Verification items for the finished model (mm, model axes). A direction names the side the tool comes from. Round coordinates to 2 decimals unless told otherwise and drop trailing zeros. Write each loop counter-clockwise with the first axis right and the second up, starting at its lowest first coordinate (ties: lowest second). Pieces come first, ordered by that corner, then holes. Notation, with made-up numbers: M -16.75,64 L 12.25,64 A4 cw 12.25,70 Z; hole C 1.5,24 d11. An arc over 180 degrees is marked long. Answer in a Markdown table with one row per item. Add a question column.
1. Set-up check for faces 1 (the flat face through (-15, 38, 0)), 2 (the cylindrical face through (-8.57, 45.39, 1.01)): record each of +Z, -Z, +X, -X, +Y, -Y from which the full face is reachable in a straight line by a thin tool's end or side.
2. Draft check along X on faces 3 (the flat face through (-31.52, 47.32, 0.99)), 4 (the cylindrical face through (-43.968, 106.947, 0.986)), 5 (the cylindrical face through (-35.71, 78.51, 1.01)). Enter one of: pulls with the +X half, pulls with the -X half, needs draft (parallel to the pull), parting line crosses it, or undercut.
3. Sectioned sample at A-A on x = -42. Record the cut outline in (y, z), plus the area to 3 significant figures.
4. Sectioned sample at C-C on z = 0.9. Count the separate pieces of the cut face and the enclosed holes in it, plus the area to 3 significant figures.
5. Material ranges on probe 1 along Y at (x, z) = (9, 0.45); probe 2 along X at (y, z) = (61, 1.9); probe 3 along Y at (x, z) = (-14.5, 1.15), recorded low to high.
6. Go/stop test with a flat-tipped pin: pin 1 Ø3.5 at (x, y) = (-17.72, 60.66) entering from +Z. Record where the tip stops, or that it passes through.
7. Sectioned sample at D-D on x = 2. Record the cut outline in (y, z), plus the area to 3 significant figures.
8. Sectioned sample at B-B on y = 72.5. Record the cut outline in (x, z).
Autodesk Inventor part; units mm, degrees
ref_plane "YZ Plane" through (0, 0, 0) normal (1, 0, 0) x (0, 1, 0)
ref_plane "XZ Plane" through (0, 0, 0) normal (0, 1, 0) x (-1, 0, 0)
ref_plane "XY Plane" through (0, 0, 0) normal (0, 0, 1) x (1, 0, 0)
sketch "Эскиз1" plane through (0, 0, 0) normal (0, 0, 1) x (1, 0, 0)
  line L0 (15, -22.25) -> (15, 22.25)
  line L1 (15, 22.25) -> (-20, 22.25)
  line L2 (-20, 22.25) -> (-20, -22.25)
  line L3 (-20, -22.25) -> (15, -22.25)
  circle A0 centre (8.763, 2.3275) radius 1.5
  circle A1 centre (8.763, 7.3275) radius 1.5
  circle A2 centre (-11.237, -7.6725) radius 1.5
  circle A3 centre (-11.237, -2.6725) radius 1.5
  circle A4 centre (8.763, -2.6725) radius 1.5
  circle A5 centre (8.763, -7.6725) radius 1.5
  circle A6 centre (-11.237, 2.3275) radius 1.5
  circle A7 centre (-11.237, 7.3275) radius 1.5
  line L4 (-25, 92.25) -> (-62.0049, 92.25)
  line L5 (-103.637, 92.25) -> (-67.893, 92.25)
  circle A8 centre (-49, 104.25) radius 1.5
  circle A9 centre (-42, 104.25) radius 1.5
  circle A10 centre (-35, 104.25) radius 1.5
  circle A11 centre (-35, 111.25) radius 1.5
  circle A12 centre (-42, 118.25) radius 1.5
  circle A13 centre (-49, 118.25) radius 1.5
  circle A14 centre (-49, 111.25) radius 1.5
  circle A15 centre (-35, 118.25) radius 1.5
  circle A16 centre (-42, 111.25) radius 1.5
  circle A17 centre (-42, 97.25) radius 1.5
  circle A18 centre (-35, 97.25) radius 1.5
  circle A19 centre (-49, 97.25) radius 1.5
  line L6 (-25, 92.25) -> (-62.0049, 92.25)
  line L7 (-25, 95.25) -> (-25, 92.25)
  line L8 (-20, 95.25) -> (-25, 95.25)
  line L9 (-20, 95.25) -> (-20, 123.25)
  line L10 (-28, 123.25) -> (-20, 123.25)
  line L11 (-28, 129.25) -> (-28, 123.25)
  line L12 (-28, 129.25) -> (-62.0049, 129.25)
  line L13 (-62.0049, 92.25) -> (-62.0049, 129.25)
  line L14 (-5.1452, 11.625) -> (-40, 100) construction
  arc A20 (-32.5697, 102.9649) -> (-47.4303, 97.0351) centre (-40, 100) ccw
  line L15 (-5.1452, 11.625) -> (-22.5726, 55.8125) construction
  arc A21 (-13.8135, 8.0713) -> (-4.3725, 15.1785) centre (-0.8009, 0.6099) ccw
  line L16 (12.7625, 7.0157) -> (-32.7662, 103.4164)
  line L17 (-47.6184, 97.5588) -> (-15.0854, -3.9674)
  point P0 (0, 0)
  point P1 (-13.8589, 33.7187)
  point P2 (-33.6095, 104.8127)
  point P3 (-34.2206, 105.5316)
  point P4 (-47.7749, 98.1155)
  point P5 (-47.5011, 97.1926)
  dimension "d0" = 8
  dimension "d1" = 95
  dimension "d2" = 100
  dimension "d3" = 40
  dimension "d4" = 15
extrude "Выдавливание1" add sketch "Эскиз1" along normal blind 2 contours L16 A21 L17 L2 L1 | L1 L2 L17 L4 L16 | L4 L17 A19 A20 A10 L16 | A20 A10 | A10 A20 | A1 | A2 | A3 | A4 | A5 | A7 | A9
sketch "Эскиз2" plane through (0, 0, 2) normal (0, 0, 1) x (1, 0, 0)
  circle A0 centre (-38.5661, 86.5462) radius 1.5
  line L0 (-47.5011, 97.1926) -> (-15.0854, -3.9674)
  circle A1 centre (-35.5146, 77.0232) radius 1.5
  circle A2 centre (-32.463, 67.5001) radius 1.5
  circle A3 centre (-29.4114, 57.9771) radius 1.5
  circle A4 centre (-26.3599, 48.4541) radius 1.5
  circle A5 centre (-23.3083, 38.9311) radius 1.5
  circle A6 centre (-20.2568, 29.408) radius 1.5
  circle A7 centre (-17.2052, 19.885) radius 1.5
  circle A8 centre (-42, 97.25) radius 1.5
  circle A9 centre (-11.237, 2.3275) radius 1.5
  point P0 (0, 0)
  dimension "d7" = 3
  dimension "d10" = 10
  dimension "d17" = 5.2562
  dimension "d18" = 5.26
extrude "Выдавливание2" cut sketch "Эскиз2" against normal blind 3 contours A0 | A1 | A2 | A3 | A4 | A5 | A6 | A7
sketch "Эскиз3" plane through (0, 0, 2) normal (0, 0, 1) x (1, 0, 0)
  circle A0 centre (-35, 97.25) radius 1.5
  line L0 (12.7625, 7.0157) -> (-32.7662, 103.4164)
  circle A1 centre (-30.5318, 87.7899) radius 1.5
  circle A2 centre (-26.2613, 78.7476) radius 1.5
  circle A3 centre (-21.9908, 69.7054) radius 1.5
  circle A4 centre (-17.7202, 60.6631) radius 1.5
  circle A5 centre (-13.4497, 51.6208) radius 1.5
  circle A6 centre (-9.1792, 42.5786) radius 1.5
  circle A7 centre (-4.9086, 33.5363) radius 1.5
  circle A8 centre (-0.6381, 24.494) radius 1.5
  point P0 (0, 0)
  dimension "d19" = 3
  dimension "d20" = 4.6533
  dimension "d21" = 4.653
  dimension "d24" = 10
extrude "Выдавливание3" cut sketch "Эскиз3" against normal blind 3 contours A1 | A2 | A3 | A4 | A5 | A6 | A7 | A8
sketch "Эскиз4" plane through (0, 0, 0) normal (0, 0, -1) x (-1, 0, 0)
  circle A0 centre (42, 97.25) radius 1.5
  circle A1 centre (35, 97.25) radius 1.5
  arc A2 (35, 97.25) -> (36.2942, 93.1949) centre (42, 97.25) ccw construction
  arc A3 (33.5, 97.25) -> (35.0715, 92.326) centre (42, 97.25) ccw
  arc A4 (36.5, 97.25) -> (37.5169, 94.0639) centre (42, 97.25) ccw
  arc A5 (36.5, 97.25) -> (33.5, 97.25) centre (35, 97.25) ccw
  arc A6 (35.0715, 92.326) -> (37.5169, 94.0639) centre (36.2942, 93.1949) ccw
  point P0 (0, 0)
extrude "Выдавливание4" cut sketch "Эскиз4" against normal blind 3 contours A4 A6 A3 A1
sketch "Эскиз5" plane through (0, 0, 2) normal (0, 0, 1) x (1, 0, 0)
  circle A0 centre (-42, 97.25) radius 1.5
  arc A1 (-35.0715, 92.326) -> (-33.5, 97.25) centre (-42, 97.25) ccw
  arc A2 (-37.5169, 94.0639) -> (-35.0715, 92.326) centre (-36.2942, 93.1949) ccw
  arc A3 (-37.5169, 94.0639) -> (-36.5, 97.25) centre (-42, 97.25) ccw
  arc A4 (-33.5, 97.25) -> (-36.5, 97.25) centre (-35, 97.25) ccw
  circle A5 centre (-11.237, 2.3275) radius 1.5
  circle A6 centre (8.763, 2.3275) radius 1.5
  arc A7 (-15.0854, -3.9674) -> (12.7625, 7.0157) centre (-0.8009, 0.6099) ccw
  line L0 (12.7625, 7.0157) -> (-32.7662, 103.4164)
  arc A8 (-32.7662, 103.4164) -> (-33.6095, 104.8127) centre (-40, 100) ccw
  arc A9 (-33.6095, 104.8127) -> (-34.2206, 105.5316) centre (-35, 104.25) ccw
  arc A10 (-34.2206, 105.5316) -> (-47.7749, 98.1155) centre (-40, 100) ccw
  arc A11 (-47.5011, 97.1926) -> (-47.7749, 98.1155) centre (-49, 97.25) ccw
  line L1 (-47.5011, 97.1926) -> (-15.0854, -3.9674)
  circle A12 centre (-17.2052, 19.885) radius 1.5
  circle A13 centre (-23.3083, 38.9311) radius 1.5
  circle A14 centre (-38.5661, 86.5462) radius 1.5
  circle A15 centre (-32.463, 67.5001) radius 1.5
  circle A16 centre (-29.4114, 57.9771) radius 1.5
  circle A17 centre (-35.5146, 77.0232) radius 1.5
  circle A18 centre (-20.2568, 29.408) radius 1.5
  circle A19 centre (-26.3599, 48.4541) radius 1.5
  circle A20 centre (-0.6381, 24.494) radius 1.5
  circle A21 centre (-26.2613, 78.7476) radius 1.5
  circle A22 centre (-4.9086, 33.5363) radius 1.5
  circle A23 centre (-13.4497, 51.6208) radius 1.5
  circle A24 centre (-17.7202, 60.6631) radius 1.5
  circle A25 centre (-9.1792, 42.5786) radius 1.5
  circle A26 centre (-30.5318, 87.7899) radius 1.5
  circle A27 centre (-21.9908, 69.7054) radius 1.5
  circle A28 centre (-23.3083, 38.9311) radius 1.5
  circle A29 centre (-9.1792, 42.5786) radius 1.5
  arc A30 (-9.149, 35.4026) -> (-9.1792, 42.5786) centre (-23.3083, 38.9311) ccw construction
  arc A31 (-7.6935, 35.0399) -> (-7.7268, 42.9535) centre (-23.3083, 38.9311) ccw
  arc A32 (-10.6045, 35.7653) -> (-10.6316, 42.2036) centre (-23.3083, 38.9311) ccw
  arc A33 (-10.6045, 35.7653) -> (-7.6935, 35.0399) centre (-9.149, 35.4026) ccw
  arc A34 (-7.7268, 42.9535) -> (-10.6316, 42.2036) centre (-9.1792, 42.5786) ccw
  arc A35 (-9.1792, 42.5786) -> (-11.0829, 46.8983) centre (-23.3083, 38.9311) ccw construction
  arc A36 (-7.7268, 42.9535) -> (-9.8263, 47.7173) centre (-23.3083, 38.9311) ccw
  arc A37 (-10.6316, 42.2036) -> (-12.3396, 46.0794) centre (-23.3083, 38.9311) ccw
  arc A38 (-10.6316, 42.2036) -> (-7.7268, 42.9535) centre (-9.1792, 42.5786) ccw
  arc A39 (-9.8263, 47.7173) -> (-12.3396, 46.0794) centre (-11.0829, 46.8983) ccw
  point P0 (0, 0)
  point P1 (-10.6316, 42.2036)
  point P2 (-10.6316, 42.2036)
  point P3 (-10.6316, 42.2036)
  point P4 (-7.7268, 42.9535)
  point P5 (-7.7268, 42.9535)
  point P6 (-7.7268, 42.9535)
extrude "Выдавливание5" cut sketch "Эскиз5" against normal blind 3 contours A25 A31 A33 A32 | A25 A37 A39 A36
properties part number "ЛЦМК000002.00.00.00.00.19 мост"
Geometry check:
| question | item | result |
|---|---|---|
| 1 | face 1 | -Z, +X, -X, +Y, -Y |
| 1 | face 2 | +Z, -Z |
| 2 | face 3 | pulls with the -X half |
| 2 | face 4 | parting line crosses it |
| 2 | face 5 | undercut |
| 3 | outline | M 80.03,0 L 95.75,0 L 95.75,2 L 80.03,2 Z; M 98.75,0 L 107.75,0 L 107.75,2 L 98.75,2 Z |
| 3 | area | 49.4 mm2 |
| 4 | separate pieces | 1 |
| 4 | enclosed holes | 20 |
| 4 | area | 2,730 mm2 |
| 5 | probe 1 | y = -10.75 to 0.85, 3.81 to 14.98 |
| 5 | probe 2 | x = -35.9 to -19.18, -16.26 to -12.73 |
| 5 | probe 3 | y = -5.5 to 50.55, 52.69 to 64.74 |
| 6 | pin 1 | stops at z = 2 |
| 7 | outline | M -14.13,0 L 29.8,0 L 29.8,2 L -14.13,2 Z |
| 7 | area | 87.9 mm2 |
| 8 | outline | M -39.59,0 L -18.16,0 L -18.16,2 L -39.59,2 Z |
